```python
from build123d import *

# Parameters (mm, degrees)
BOSS_EXTRUDE1_DEPTH            = 1
BOSS_EXTRUDE2_DEPTH            = 2
BOSS_EXTRUDE3_DEPTH            = 5
BOSS_EXTRUDE4_DEPTH            = 13
CUT_EXTRUDE1_REACH             = 99.519
CUT_EXTRUDE1_DIRECTION_2_REACH = 99.519
BOSS_EXTRUDE5_DEPTH            = 0.5
F_10_0_1935_DIAMETER_HOLE1_D   = 4.9149


with BuildPart() as part:
    # Sketch1 → Boss-Extrude1 (new body)
    with BuildSketch(Plane.XY):
        with BuildLine():
            Line((-14.5, 27.975526805), (-14.5, -38.491666667))
            Line((-14.5, -38.491666667), (-10, -38.491666667))
            ThreePointArc((-10, -38.491666667), (0, -33.491666667), (10, -38.491666667))
            Line((10, -38.491666667), (14.5, -38.491666667))
            Line((14.5, -38.491666667), (14.5, 27.975526805))
            Line((14.5, 27.975526805), (14.5, 31.314135298))
            ThreePointArc((14.5, 31.314135298), (0, 34.508333333), (-14.5, 31.314135298))
            Line((-14.5, 31.314135298), (-14.5, 27.975526805))
        make_face()
        with BuildLine():
            Line((-11.5, -21.491666667), (-11.5, 22.592219961))
            ThreePointArc((-11.5, 22.592219961), (-11.165907115, 23.698905773), (-10.275246515, 24.435855728))
            ThreePointArc((-10.275246515, 24.435855728), (0, 26.508333333), (10.275246515, 24.435855728))
            ThreePointArc((10.275246515, 24.435855728), (11.165907115, 23.698905773), (11.5, 22.592219961))
            Line((11.5, 22.592219961), (11.5, -21.491666667))
            ThreePointArc((11.5, -21.491666667), (10.914213562, -22.905880229), (9.5, -23.491666667))
            Line((9.5, -23.491666667), (-9.5, -23.491666667))
            ThreePointArc((-9.5, -23.491666667), (-10.914213562, -22.905880229), (-11.5, -21.491666667))
        make_face(mode=Mode.SUBTRACT)
    extrude(amount=BOSS_EXTRUDE1_DEPTH)

    # Sketch1_3 → Boss-Extrude2 (add)
    with BuildSketch(Plane.XY):
        with BuildLine():
            ThreePointArc((-27.5, -38.491666667), (-26.914213562, -39.905880229), (-25.5, -40.491666667))
            Line((-25.5, -40.491666667), (-14.5, -40.491666667))
            Line((-14.5, -40.491666667), (-14.5, -38.491666667))
            Line((-14.5, -38.491666667), (-14.5, 27.975526805))
            ThreePointArc((-14.5, 27.975526805), (-21.72589695, 22.822477992), (-27.228227719, 15.858868663))
            ThreePointArc((-27.228227719, 15.858868663), (-27.430861911, 15.373593751), (-27.5, 14.85227592))
            Line((-27.5, 14.85227592), (-27.5, 4.508333333))
            Line((-27.5, 4.508333333), (-21.5, 4.508333333))
            Line((-21.5, 4.508333333), (-21.5, -10.491666667))
            Line((-21.5, -10.491666667), (-27.5, -10.491666667))
            Line((-27.5, -10.491666667), (-27.5, -38.491666667))
        make_face()
        with BuildLine():
            Line((14.5, -40.491666667), (25.5, -40.491666667))
            ThreePointArc((25.5, -40.491666667), (26.914213562, -39.905880229), (27.5, -38.491666667))
            Line((27.5, -38.491666667), (27.5, -10.491666667))
            Line((27.5, -10.491666667), (21.5, -10.491666667))
            Line((21.5, -10.491666667), (21.5, 4.508333333))
            Line((21.5, 4.508333333), (27.5, 4.508333333))
            Line((27.5, 4.508333333), (27.5, 14.85227592))
            ThreePointArc((27.5, 14.85227592), (27.430861911, 15.373593751), (27.228227719, 15.858868663))
            ThreePointArc((27.228227719, 15.858868663), (21.72589695, 22.822477992), (14.5, 27.975526805))
            Line((14.5, 27.975526805), (14.5, -38.491666667))
            Line((14.5, -38.491666667), (14.5, -40.491666667))
        make_face()
    extrude(amount=BOSS_EXTRUDE2_DEPTH)

    # Sketch1_5 → Boss-Extrude3 (add)
    with BuildSketch(Plane.XY):
        with BuildLine():
            ThreePointArc((29.5, 21.508333333), (0, 36.508333333), (-29.5, 21.508333333))
            Line((-29.5, 21.508333333), (-29.5, -38.491666667))
            Line((-29.5, -38.491666667), (-30.323529412, -40.491666667))
            Line((-30.323529412, -40.491666667), (-25.5, -40.491666667))
            ThreePointArc((-25.5, -40.491666667), (-26.914213562, -39.905880229), (-27.5, -38.491666667))
            Line((-27.5, -38.491666667), (-27.5, -10.491666667))
            Line((-27.5, -10.491666667), (-27.5, 4.508333333))
            Line((-27.5, 4.508333333), (-27.5, 14.85227592))
            ThreePointArc((-27.5, 14.85227592), (-27.430861911, 15.373593751), (-27.228227719, 15.858868663))
            ThreePointArc((-27.228227719, 15.858868663), (-21.72589695, 22.822477992), (-14.5, 27.975526805))
            Line((-14.5, 27.975526805), (-14.5, 31.314135298))
            ThreePointArc((-14.5, 31.314135298), (0, 34.508333333), (14.5, 31.314135298))
            Line((14.5, 31.314135298), (14.5, 27.975526805))
            ThreePointArc((14.5, 27.975526805), (21.72589695, 22.822477992), (27.228227719, 15.858868663))
            ThreePointArc((27.228227719, 15.858868663), (27.430861911, 15.373593751), (27.5, 14.85227592))
            Line((27.5, 14.85227592), (27.5, 4.508333333))
            Line((27.5, 4.508333333), (27.5, -10.491666667))
            Line((27.5, -10.491666667), (27.5, -38.491666667))
            ThreePointArc((27.5, -38.491666667), (26.914213562, -39.905880229), (25.5, -40.491666667))
            Line((25.5, -40.491666667), (30.323529412, -40.491666667))
            Line((30.323529412, -40.491666667), (29.5, -38.491666667))
            Line((29.5, -38.491666667), (29.5, 21.508333333))
        make_face()
    extrude(amount=BOSS_EXTRUDE3_DEPTH)

    # Sketch1_6 → Boss-Extrude4 (add)
    with BuildSketch(Plane.XY):
        with BuildLine():
            Line((-25.5, -40.491666667), (-30.323529412, -40.491666667))
            Line((-30.323529412, -40.491666667), (-36.5, -55.491666667))
            Line((-36.5, -55.491666667), (-36.5, -71.491666667))
            ThreePointArc((-36.5, -71.491666667), (-28.968061706, -81.149889898), (-20, -89.491666667))
            ThreePointArc((-20, -89.491666667), (0, -86.951333591), (20, -89.491666667))
            ThreePointArc((20, -89.491666667), (28.968061706, -81.149889898), (36.5, -71.491666667))
            Line((36.5, -71.491666667), (36.5, -55.491666667))
            Line((36.5, -55.491666667), (30.323529412, -40.491666667))
            Line((30.323529412, -40.491666667), (25.5, -40.491666667))
            Line((25.5, -40.491666667), (14.5, -40.491666667))
            Line((14.5, -40.491666667), (14.5, -41.491666667))
            Line((14.5, -41.491666667), (-14.5, -41.491666667))
            Line((-14.5, -41.491666667), (-14.5, -40.491666667))
            Line((-14.5, -40.491666667), (-25.5, -40.491666667))
        make_face()
    extrude(amount=BOSS_EXTRUDE4_DEPTH)

    # Sketch2 → Cut-Extrude1 (cut, up to next)
    with BuildSketch(Plane(origin=(0, 0, 0), x_dir=(0, 0, -1), z_dir=(1, 0, 0)), mode=Mode.PRIVATE) as cut_extrude1_sk1:
        Polygon((-5, -40.491666667), (-13, -55.491666667), (-13, -40.491666667), align=None)
    cut_extrude1_tool1 = extrude(cut_extrude1_sk1.sketch, amount=-CUT_EXTRUDE1_REACH, mode=Mode.PRIVATE) & part.part
    # Sketch2 → Cut-Extrude1 (cut, up to next)
    with BuildSketch(Plane(origin=(0, 0, 0), x_dir=(0, 0, -1), z_dir=(1, 0, 0)), mode=Mode.PRIVATE) as cut_extrude1_sk2:
        Polygon((-13, -71.491666667), (0, -89.491666667), (-13, -89.491666667), align=None)
    cut_extrude1_tool2 = extrude(cut_extrude1_sk2.sketch, amount=-CUT_EXTRUDE1_REACH, mode=Mode.PRIVATE) & part.part
    add(cut_extrude1_tool1.solids().sort_by_distance((0, -45.491667, 10.333333))[0], mode=Mode.SUBTRACT)
    add(cut_extrude1_tool2.solids().sort_by_distance((0, -83.491667, 8.666667))[0], mode=Mode.SUBTRACT)

    # Sketch2 → Cut-Extrude1 direction 2 (cut, up to next)
    with BuildSketch(Plane(origin=(0, 0, 0), x_dir=(0, 0, -1), z_dir=(1, 0, 0)), mode=Mode.PRIVATE) as cut_extrude1_direction_2_sk1:
        Polygon((-5, -40.491666667), (-13, -55.491666667), (-13, -40.491666667), align=None)
    cut_extrude1_direction_2_tool1 = extrude(cut_extrude1_direction_2_sk1.sketch, amount=CUT_EXTRUDE1_DIRECTION_2_REACH, mode=Mode.PRIVATE) & part.part
    # Sketch2 → Cut-Extrude1 direction 2 (cut, up to next)
    with BuildSketch(Plane(origin=(0, 0, 0), x_dir=(0, 0, -1), z_dir=(1, 0, 0)), mode=Mode.PRIVATE) as cut_extrude1_direction_2_sk2:
        Polygon((-13, -71.491666667), (0, -89.491666667), (-13, -89.491666667), align=None)
    cut_extrude1_direction_2_tool2 = extrude(cut_extrude1_direction_2_sk2.sketch, amount=CUT_EXTRUDE1_DIRECTION_2_REACH, mode=Mode.PRIVATE) & part.part
    add(cut_extrude1_direction_2_tool1.solids().sort_by_distance((0, -45.491667, 10.333333))[0], mode=Mode.SUBTRACT)
    add(cut_extrude1_direction_2_tool2.solids().sort_by_distance((0, -83.491667, 8.666667))[0], mode=Mode.SUBTRACT)

    # Sketch3 → Boss-Extrude5 (add)
    with BuildSketch(Plane.XY.offset(13)):
        with BuildLine():
            Line((-33.5, -61.491666667), (-33.5, -65.491666667))
            ThreePointArc((-33.5, -65.491666667), (-32.621320344, -67.61298701), (-30.5, -68.491666667))
            Line((-30.5, -68.491666667), (30.5, -68.491666667))
            ThreePointArc((30.5, -68.491666667), (32.621320344, -67.61298701), (33.5, -65.491666667))
            Line((33.5, -65.491666667), (33.5, -61.491666667))
            ThreePointArc((33.5, -61.491666667), (32.621320344, -59.370346323), (30.5, -58.491666667))
            Line((30.5, -58.491666667), (-30.5, -58.491666667))
            ThreePointArc((-30.5, -58.491666667), (-32.621320344, -59.370346323), (-33.5, -61.491666667))
        make_face()
    extrude(amount=BOSS_EXTRUDE5_DEPTH)

    # 10 _0.1935_ Diameter Hole1 (through all)
    with Locations(Plane.XY.offset(2)):
        with Locations((19.5, -32.491666667), (-19.5, -32.491666667), (-19.5, 9.508333333), (19.5, 9.508333333)):
            Hole(F_10_0_1935_DIAMETER_HOLE1_D / 2)


solid = part.part
```
Geometry check sheet. Reference: the model listing, model coordinates, mm. A direction names the side the tool comes from. Coordinates: 2 decimals unless noted, no trailing zeros. Order: outer loops, then holes, each group sorted by start corner. A loop starts at its lowest first (then second) coordinate and runs counter-clockwise, first axis right, second up. Notation, with made-up numbers: M -30,17 L -14,17 A14 cw -14,44 Z; hole C -12.75,22.25 d1. An arc over 180 degrees is marked long. Answer as a JSON object with one key per item and string values.
Q1. Release check for a two-part mould opening along X. For faces 1 (the flat face through (27.5, -11, 3)), 2 (the flat face through (-21, -13, 2)), 3 (the flat face through (-29.5, -8, 2)), 4 (the flat face through (-18, 27, 5)) record: released by +X, released by -X, zero draft, split by the parting line, or undercut.
Results are:
{"face 1": "undercut", "face 2": "undercut", "face 3": "released by -X", "face 4": "zero draft"}
Q2. Depth check by flat-ended pin: pin 1 Ø8 at (x, z) = (11, 12) entering from -Y; pin 2 Ø3 at (y, z) = (-13, 3.5) entering from -X; pin 3 Ø4 at (x, z) = (19.5, 5.5) entering from +Y; pin 4 Ø3 at (x, y) = (-16.5, 4.5) entering from -Z. Enter the tip coordinate at first touch or a pass-through.
Results are:
{"pin 1": "stops at y = -78.41", "pin 2": "stops at x = -29.5", "pin 3": "stops at y = 32.01", "pin 4": "stops at z = 0"}
Q3. Cross-section at A-A on x = 2. Record the cut outline in (y, z).
Results are:
{"outline": "M -86.98,0 L -41.49,0 L -41.49,5.53 L -55.49,13 L -58.49,13 L -58.49,13.5 L -68.49,13.5 L -68.49,13 L -71.49,13 L -86.98,1.82 Z; M -33.65,0 L -23.49,0 L -23.49,1 L -33.65,1 Z; M 26.43,0 L 36.45,0 L 36.45,5 L 34.45,5 L 34.45,1 L 26.43,1 Z"}
Q4. Tool access check on faces 5 (the cylindrical face through (-0.21, 34.508, 2.972)), 6 (the cylindrical face through (-32.6, -59.35, 13.25)), 7 (the cylindrical face through (32.598, -67.636, 13.246)). Record the directions out of +Z, -Z, +X, -X, +Y, -Y that give a thin tool (end or side, any length) a straight path to the whole face; none if there is none.
Results are:
{"face 5": "+Z", "face 6": "+Z, -X, +Y", "face 7": "+Z, +X, -Y"}
Q5. Scan lines: line 1 (Y direction, x = -19.5, z = 0.65); line 2 (X direction, y = 10.5, z = 2.5); line 3 (Y direction, x = -19.5, z = 0.5). Record each from-to range of solid material in increasing order.
Results are:
{"line 1": "y = -88.59 to -34.95, -30.03 to 7.05, 11.97 to 30.86", "line 2": "x = -29.5 to -27.5, 27.5 to 29.5", "line 3": "y = -88.8 to -34.95, -30.03 to 7.05, 11.97 to 30.86"}
Q6. Cross-section at B-B on z = 8.25. Record the cut outline in (x, y), and give its area (3 significant figures).
Results are:
{"outline": "M -36.5,-71.49 A77 ccw -31.65,-78.07 L 31.65,-78.07 A77 ccw 36.5,-71.49 L 36.5,-55.49 L 32.83,-46.59 L -32.83,-46.59 L -36.5,-55.49 Z", "area": "2,230 mm²"}
